Here's the drawing with two shaded views (mm, measured from the low corner). I have some questions. Give positions to 0.01 mm unless a question says otherwise; leave off trailing zeros. Loops run counter-clockwise (first coordinate to the right, second up) from the corner with the lowest first, then second, coordinate; pieces in that order, holes last. Notation, with made-up numbers: (21.25, 65.5) -> (29.25, 65.5) arc R7 cw to (29.25, 70.5) -> close; hole circle Ø4 at (55, 89). An arc over 180 degrees is marked (long way). Answer in a Markdown table with one row per item. Add a question column.
Item 1: If we section it at B-B (x = 19.25): Write out the boundary of the cut face in (y, z) (1 decimal).
Item 2: If I drill on line 1 (X direction, y = 0.5, z = 0.2); line 2 (Y direction, x = 12.25, z = 0.3) (1 decimal); line 3 (X direction, y = 4, z = 0.35), over which ranges is the centre line in solid material (lowest first)?
Item 3: If we section it at C-C (y = 9.75): Write out the boundary of the cut face in (x, z).
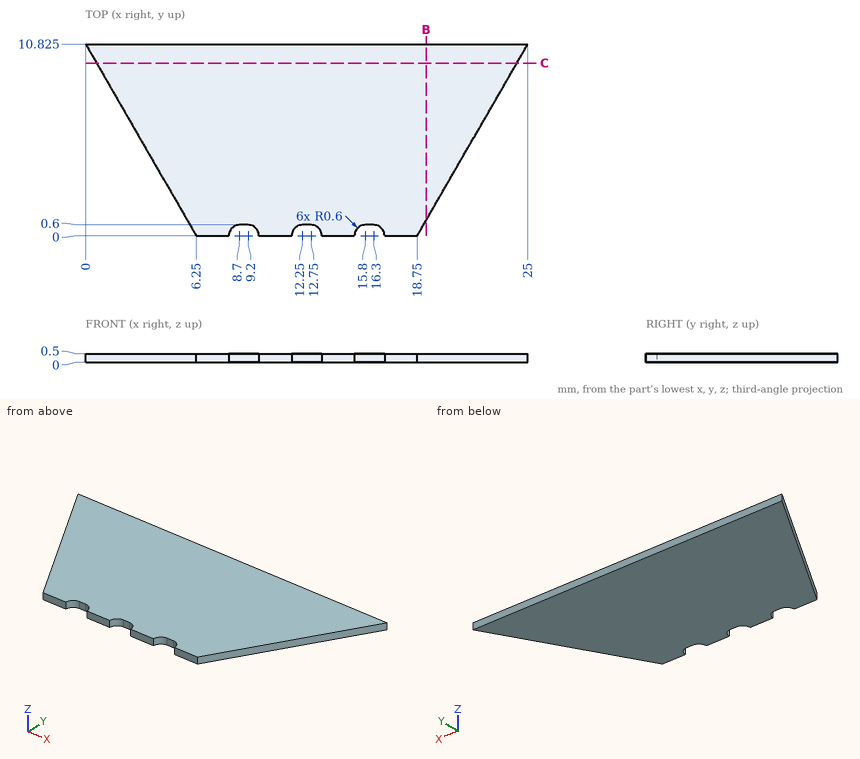
Recorded:
| question | item | result |
|---|---|---|
| 1 | outline | (0.9, 0) -> (10.8, 0) -> (10.8, 0.5) -> (0.9, 0.5) -> close |
| 2 | line 1 | x = 5.96 to 8.37, 9.53 to 11.92, 13.08 to 15.47, 16.63 to 19.04 |
| 2 | line 2 | y = 0.6 to 10.8 |
| 2 | line 3 | x = 3.94 to 21.06 |
| 3 | outline | (0.62, 0) -> (24.38, 0) -> (24.38, 0.5) -> (0.62, 0.5) -> close |
